from build123d import *

# Parameters (mm, degrees)
SKETCH1_R            = 3.96875
BOSS_EXTRUDE2_DEPTH  = 6.35
BOSS_EXTRUDE3_DEPTH  = 12.7
SKETCH3_R            = 15.7226
BOSS_EXTRUDE4_DEPTH  = 25.4
SKETCH4_R            = 3.96875
BOSS_EXTRUDE5_DEPTH  = 6.35
BOSS_EXTRUDE6_DEPTH  = 12.7
SKETCH6_R            = 9.0805
BOSS_EXTRUDE8_DEPTH  = 12.8778
SKETCH8_W            = 7.8486
SKETCH8_H            = 8.0772
SKETCH8_W_2          = 8.0772
SKETCH8_H_2          = 7.8486
BOSS_EXTRUDE9_DEPTH  = 2.9464
BOSS_EXTRUDE10_START = -2.9464
BOSS_EXTRUDE10_DEPTH = 2.9464


with BuildPart() as part:
    # Sketch1 → Boss-Extrude2 (new body)
    with BuildSketch(Plane(origin=(0, 0, 0), x_dir=(0, 0, -1), z_dir=(1, 0, 0))):
        with BuildLine():
            Line((-19.834703053, 12.065523939), (-14.896576623, 5.029130709))
            ThreePointArc((-14.896576623, 5.029130709), (-15.7226, 0), (-14.896576623, -5.029130709))
            Line((-14.896576623, -5.029130709), (-19.834703053, -12.065523939))
            ThreePointArc((-19.834703053, -12.065523939), (-19.086763334, -19.086763334), (-12.065523939, -19.834703053))
            Line((-12.065523939, -19.834703053), (-5.029130709, -14.896576623))
            ThreePointArc((-5.029130709, -14.896576623), (0, -15.7226), (5.029130709, -14.896576623))
            Line((5.029130709, -14.896576623), (12.065523939, -19.834703053))
            ThreePointArc((12.065523939, -19.834703053), (19.086763334, -19.086763334), (19.834703053, -12.065523939))
            Line((19.834703053, -12.065523939), (14.896576623, -5.029130709))
            ThreePointArc((14.896576623, -5.029130709), (15.7226, 0), (14.896576623, 5.029130709))
            Line((14.896576623, 5.029130709), (19.834703053, 12.065523939))
            ThreePointArc((19.834703053, 12.065523939), (19.086763334, 19.086763334), (12.065523939, 19.834703053))
            Line((12.065523939, 19.834703053), (5.029130709, 14.896576623))
            ThreePointArc((5.029130709, 14.896576623), (0, 15.7226), (-5.029130709, 14.896576623))
            Line((-5.029130709, 14.896576623), (-12.065523939, 19.834703053))
            ThreePointArc((-12.065523939, 19.834703053), (-19.086763334, 19.086763334), (-19.834703053, 12.065523939))
        make_face()
        with Locations((-15.113, 15.113)):
            Circle(SKETCH1_R, mode=Mode.SUBTRACT)
        with Locations(Location((15.113, 15.113, 0), (0, 0, 180))):
            Circle(SKETCH1_R, mode=Mode.SUBTRACT)
        with Locations((15.113, -15.113)):
            Circle(SKETCH1_R, mode=Mode.SUBTRACT)
        with Locations(Location((-15.113, -15.113, 0), (0, 0, 180))):
            Circle(SKETCH1_R, mode=Mode.SUBTRACT)
    extrude(amount=BOSS_EXTRUDE2_DEPTH)

    # Sketch2 → Boss-Extrude3 (add)
    with BuildSketch(Plane.ZY):
        Polygon((13.680992893, 5.666852803), (13.680992893, -5.666852803), (5.666852803, -13.680992893), (-5.666852803, -13.680992893), (-13.680992893, -5.666852803), (-13.680992893, 5.666852803), (-5.666852803, 13.680992893), (5.666852803, 13.680992893), align=None)
    extrude(amount=BOSS_EXTRUDE3_DEPTH)

    # Sketch3 → Boss-Extrude4 (add)
    with BuildSketch(Plane(origin=(6.35, 0, 0), x_dir=(0, 0, -1), z_dir=(1, 0, 0))):
        with Locations(Location((0, 0, 0), (0, 0, 161.345157372))):
            Circle(SKETCH3_R)
    extrude(amount=BOSS_EXTRUDE4_DEPTH)

    # Sketch4 → Boss-Extrude5 (add)
    with BuildSketch(Plane(origin=(31.75, 0, 0), x_dir=(0, 0, -1), z_dir=(1, 0, 0))):
        with BuildLine():
            Line((-19.834703053, 12.065523939), (-14.896576623, 5.029130709))
            ThreePointArc((-14.896576623, 5.029130709), (-15.7226, 0), (-14.896576623, -5.029130709))
            Line((-14.896576623, -5.029130709), (-19.834703053, -12.065523939))
            ThreePointArc((-19.834703053, -12.065523939), (-19.086763334, -19.086763334), (-12.065523939, -19.834703053))
            Line((-12.065523939, -19.834703053), (-5.029130709, -14.896576623))
            ThreePointArc((-5.029130709, -14.896576623), (0, -15.7226), (5.029130709, -14.896576623))
            Line((5.029130709, -14.896576623), (12.065523939, -19.834703053))
            ThreePointArc((12.065523939, -19.834703053), (19.086763334, -19.086763334), (19.834703053, -12.065523939))
            Line((19.834703053, -12.065523939), (14.896576623, -5.029130709))
            ThreePointArc((14.896576623, -5.029130709), (15.7226, 0), (14.896576623, 5.029130709))
            Line((14.896576623, 5.029130709), (19.834703053, 12.065523939))
            ThreePointArc((19.834703053, 12.065523939), (19.086763334, 19.086763334), (12.065523939, 19.834703053))
            Line((12.065523939, 19.834703053), (5.029130709, 14.896576623))
            ThreePointArc((5.029130709, 14.896576623), (0, 15.7226), (-5.029130709, 14.896576623))
            Line((-5.029130709, 14.896576623), (-12.065523939, 19.834703053))
            ThreePointArc((-12.065523939, 19.834703053), (-19.086763334, 19.086763334), (-19.834703053, 12.065523939))
        make_face()
        with Locations((-15.113, 15.113)):
            Circle(SKETCH4_R, mode=Mode.SUBTRACT)
        with Locations(Location((15.113, 15.113, 0), (0, 0, 180))):
            Circle(SKETCH4_R, mode=Mode.SUBTRACT)
        with Locations((15.113, -15.113)):
            Circle(SKETCH4_R, mode=Mode.SUBTRACT)
        with Locations(Location((-15.113, -15.113, 0), (0, 0, 180))):
            Circle(SKETCH4_R, mode=Mode.SUBTRACT)
    extrude(amount=BOSS_EXTRUDE5_DEPTH)

    # Sketch5 → Boss-Extrude6 (add)
    with BuildSketch(Plane(origin=(38.1, 0, 0), x_dir=(0, 0, -1), z_dir=(1, 0, 0))):
        Polygon((13.680992893, 5.666852803), (13.680992893, -5.666852803), (5.666852803, -13.680992893), (-5.666852803, -13.680992893), (-13.680992893, -5.666852803), (-13.680992893, 5.666852803), (-5.666852803, 13.680992893), (5.666852803, 13.680992893), align=None)
    extrude(amount=BOSS_EXTRUDE6_DEPTH)

    # Sketch6 → Boss-Extrude8 (add)
    with BuildSketch(Plane(origin=(0, 13.680992893, 0), x_dir=(1, 0, 0), z_dir=(0, 1, 0))):
        with Locations(Location((19.05, 0.284018035, 0), (0, 0, 55.282753466))):
            Circle(SKETCH6_R)
    extrude(amount=BOSS_EXTRUDE8_DEPTH)

    # Sketch8 → Boss-Extrude9 (add)
    with BuildSketch(Plane(origin=(0, 26.558792893, 0), x_dir=(1, 0, 0), z_dir=(0, 1, 0))):
        with Locations((19.05, 10.202718035)):
            Rectangle(SKETCH8_W, SKETCH8_H)
        with Locations((9.1313, 0.284018035)):
            Rectangle(SKETCH8_W_2, SKETCH8_H_2)
    extrude(amount=-BOSS_EXTRUDE9_DEPTH)

    # Sketch10 → Boss-Extrude10 (add)
    with BuildSketch(Plane(origin=(0, 26.558792893, 0), x_dir=(1, 0, 0), z_dir=(0, 1, 0)).offset(BOSS_EXTRUDE10_START)):
        with BuildLine():
            Line((24.7523, 7.350789218), (31.6103, 7.350789218))
            Line((31.6103, 7.350789218), (31.6103, 5.064789218))
            Line((31.6103, 5.064789218), (28.1305, 5.064789218))
            Line((28.1305, 5.064789218), (28.1305, 0.284018035))
            ThreePointArc((28.1305, 0.284018035), (23.784459378, -7.464554392), (14.90647607, -7.795999892))
            Line((14.90647607, -7.795999892), (14.90647607, -12.140453608))
            Line((14.90647607, -12.140453608), (12.11247607, -12.140453608))
            Line((12.11247607, -12.140453608), (11.743935589, -5.108282316))
            ThreePointArc((11.743935589, -5.108282316), (12.769066077, 6.841864427), (24.7523, 7.350789218))
        make_face()
    extrude(amount=BOSS_EXTRUDE10_DEPTH)


solid = part.part
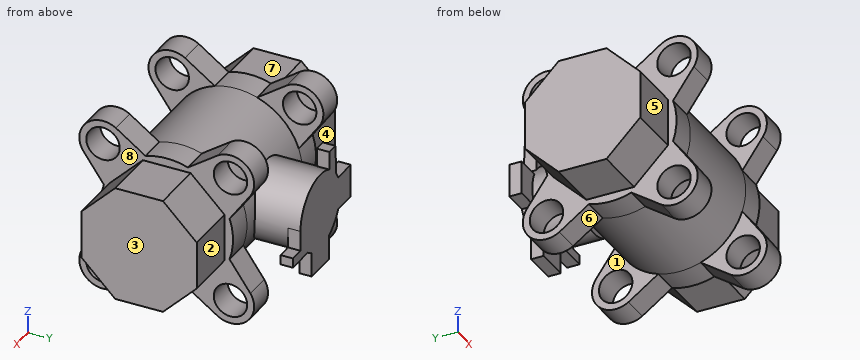
Check sheet for the modelled part. Datum: model origin and axes. Units: mm. Face numbers are marked on the shaded views. A direction names the side the tool comes from. Round coordinates to 2 decimals unless told otherwise and drop trailing zeros. Order: outer loops, then holes, each group sorted by start corner. A loop starts at its lowest first (then second) coordinate and runs counter-clockwise, first axis right, second up.
Q1. Scan lines: L1, parallel to Z at x = 5, y = -16; L2, parallel to Y at x = 16, z = -0.5; L3, parallel to X at y = 15, z = 9.5. Record each from-to range of solid material in increasing order.
Filled sheet:
L1: z = -20.66 to -18.98, -11.24 to -6.6, 6.6 to 11.24, 18.98 to 20.66
L2: y = -15.71 to 26.56
L3: x = 0 to 6.35, 31.75 to 38.1
Q2. Cross-section at D-D, the plane x = 34. Enter the section's corners in (y, z).
Filled sheet:
outline: (-19.83, -12.07) arc R5.62 ccw to (-12.07, -19.83) - (-5.03, -14.9) arc R15.72 ccw to (5.03, -14.9) - (12.07, -19.83) arc R5.62 ccw to (19.83, -12.07) - (14.9, -5.03) arc R15.72 ccw to (14.9, 5.03) - (19.83, 12.07) arc R5.62 ccw to (12.07, 19.83) - (5.03, 14.9) arc R15.72 ccw to (-5.03, 14.9) - (-12.07, 19.83) arc R5.62 ccw to (-19.83, 12.07) - (-14.9, 5.03) arc R15.72 ccw to (-14.9, -5.03) - close; hole circle Ø7.94 at (-15.11, -15.11); hole circle Ø7.94 at (-15.11, 15.11); hole circle Ø7.94 at (15.11, -15.11); hole circle Ø7.94 at (15.11, 15.11)
Q3. Draft check along X on the marked faces 1, 2 and 3. Enter one of: pulls with the +X half, pulls with the -X half, needs draft (parallel to the pull), parting line crosses it, or undercut.
Filled sheet:
face 1: undercut
face 2: needs draft
face 3: pulls with the +X half
Q4. Set-up check for the marked faces 4, 5, 6, 7 and 8: record each of +Z, -Z, +X, -X, +Y, -Y from which the full face is reachable in a straight line by a thin tool's end or side.
Filled sheet:
face 4: +Z, -Z, -X, +Y
face 5: +Z, -Z, -X, -Y
face 6: -Z, +X, -X
face 7: +Z, -X, +Y, -Y
face 8: +X
Q5. Cross-section at A-A, the plane y = -17. Give the number of separate pieces and of enclosed holes in the cut face, plus the area to 3 significant figures.
Filled sheet:
separate pieces: 8
enclosed holes: 0
area: 137 mm2
Q6. Depth check by flat-ended pin: P1, Ø1, axis at x = 36.5, z = -1, coming from the +Y side; P2, Ø3.5, axis at x = 46, z = -1, coming from the -Y side; P3, Ø3.5, axis at x = 14, z = 7, coming from the -Y side. Enter the tip coordinate at first touch or a pass-through.
Filled sheet:
P1: stops at y = 15.71
P2: stops at y = -13.68
P3: stops at y = -14.82
Q7. Cross-section at C-C, the plane x = 19.05. Enter the section's corners in (y, z).
Filled sheet:
outline: (13.68, -9.36) - (23.61, -9.36) - (23.61, -14.24) - (26.56, -14.24) - (26.56, 8.8) - (13.68, 8.8) - (13.68, 7.75) arc R15.72 ccw (long way) to (13.68, -7.75) - close
